```python
from build123d import *

# Parameters (mm, degrees)
BOSS_EXTRUDE1_DEPTH = 2.54
SKETCH3_R           = 2.413
CUT_EXTRUDE1_DEPTH  = 70.828376229


with BuildPart() as part:
    # Sketch1 → Boss-Extrude1 (new body)
    with BuildSketch(Plane.XY):
        Polygon((-31.75, 28.792017296), (31.75, 28.792017296), (35.44828546, -13.479578937), (19.05, -60.107982704), (-19.05, -60.107982704), (-35.44828546, -13.479578937), align=None)
    extrude(amount=BOSS_EXTRUDE1_DEPTH)

    # Sketch3 → Cut-Extrude1 (cut, through all)
    with BuildSketch(Plane(origin=(0, 0, 0), x_dir=(-1, 0, 0), z_dir=(0, 0, -1))):
        with Locations((11.43, -52.487982704)):
            Circle(SKETCH3_R)
        with Locations((-11.43, -52.487982704)):
            Circle(SKETCH3_R)
        with Locations((21.59, -13.479578937)):
            Circle(SKETCH3_R)
        with Locations((-21.59, -13.479578937)):
            Circle(SKETCH3_R)
    extrude(amount=-CUT_EXTRUDE1_DEPTH, mode=Mode.SUBTRACT)


solid = part.part
```
Geometry: final body of the model. Coordinates: model frame, mm. Give positions to 0.01 mm unless a question says otherwise; leave off trailing zeros. Loops run counter-clockwise (first coordinate to the right, second up) from the corner with the lowest first, then second, coordinate; pieces in that order, holes last. Notation, with made-up numbers: (-5.75, 5) -> (17.25, 5) arc R20 ccw to (17.25, 37) -> close; hole circle Ø8 at (56, 13). An arc over 180 degrees is marked (long way). Use one line per item in the form item = value.
Item 1: Pin query (flat end, axial travel): P1, Ø4, axis at x = 21.59, y = -13.48, coming from the -Z side. Return the tip coordinate at first contact, or that it passes through.
A:
P1 = through
Item 2: Section query A-A on x = -11.43. Output: boundary loops of the cut face in (y, z).
A:
outline = (-60.11, 0) -> (-54.9, 0) -> (-54.9, 2.54) -> (-60.11, 2.54) -> close; (-50.07, 0) -> (28.79, 0) -> (28.79, 2.54) -> (-50.07, 2.54) -> close
Item 3: Line query: probe 1 along Y at (x, z) = (-11.43, 1.2); probe 2 along X at (y, z) = (-13, 1.35); probe 3 along X at (y, z) = (10, 1.95). Output: solid intervals per line, ascending.
A:
probe_1 = -60.11 to -54.9, -50.07 to 28.79
probe_2 = -35.41 to -23.95, -19.23 to 19.23, 23.95 to 35.41
probe_3 = -33.39 to 33.39
Item 4: Section query B-B on z = 1.05. Output: boundary loops of the cut face in (x, y).
A:
outline = (-35.45, -13.48) -> (-19.05, -60.11) -> (19.05, -60.11) -> (35.45, -13.48) -> (31.75, 28.79) -> (-31.75, 28.79) -> close; hole circle Ø4.83 at (-21.59, -13.48); hole circle Ø4.83 at (-11.43, -52.49); hole circle Ø4.83 at (11.43, -52.49); hole circle Ø4.83 at (21.59, -13.48)
Item 5: Section query D-D on y = -4. Output: boundary loops of the cut face in (x, z).
A:
outline = (-34.62, 0) -> (34.62, 0) -> (34.62, 2.54) -> (-34.62, 2.54) -> close
Item 6: Draft query along Y for faces 1 (the face through (-27.134, -37.12, 1.252)), 2 (the face through (24, -13.4, 1.3)), 3 (the face through (-11.116, -50.096, 1.252)), 4 (the face through (33.573, 7.952, 1.252)). Return one class per face: pulls with the +Y half, pulls with the -Y half, needs draft (parallel to the pull), parting line crosses it, or undercut.
A:
face_1 = pulls with the -Y half
face_2 = undercut
face_3 = undercut
face_4 = pulls with the +Y half
Item 7: Section query C-C on x = -21.59. Output: boundary loops of the cut face in (y, z).
A:
outline = (-52.89, 0) -> (-15.89, 0) -> (-15.89, 2.54) -> (-52.89, 2.54) -> close; (-11.07, 0) -> (28.79, 0) -> (28.79, 2.54) -> (-11.07, 2.54) -> close
